The model under review builds one solid part; all positions refer to its coordinate system, in mm. Round coordinates to 2 decimals unless told otherwise and drop trailing zeros. Write each loop counter-clockwise with the first axis right and the second up, starting at its lowest first coordinate (ties: lowest second). Pieces come first, ordered by that corner, then holes. Notation, with made-up numbers: M 60.25,-7 L 92.25,-7 A29 ccw 92.25,27 Z; hole C 68.5,-27.75 d1. An arc over 180 degrees is marked long. One line per item, written item: value. Start each with the question number.
1) For P1, Ø2, axis at y = -366, z = 3, coming from the +X side, flat-tipped, find the tip position at first contact; note if it passes through.
2) Take a section at B-B, the plane z = 2.5. State how many separate pieces and enclosed holes the cut face has, and give its area (3 significant figures).
3) Take a section at A-A, the plane y = -298.5. Write out the cut boundary in (x, z), and give its area (3 significant figures).
4) Wall thickness on probe 1 along Y at (x, z) = (222.25, 3); probe 2 along Y at (x, z) = (0, 5.25); probe 3 along Y at (x, z) = (444.5, 2): over which ranges is each line inside the solid? List them lowest first.
from build123d import *

# Parameters (mm, degrees)
BOSS_EXTRUDE1_DEPTH = 6.35
SKETCH2_R           = 3.3655
CUT_EXTRUDE1_DEPTH  = 7.35
SKETCH3_R           = 3.3655
CUT_EXTRUDE2_DEPTH  = 7.35
SKETCH5_W           = 38.1
SKETCH5_H           = 82.55
CUT_EXTRUDE3_DEPTH  = 7.35
FILLET1_R           = 6.35


with BuildPart() as part:
    # Sketch1 → Boss-Extrude1 (new body)
    with BuildSketch(Plane.XY):
        Polygon((-508, 0), (508, 0), (508, -184.15), (234.95, -184.15), (234.95, -457.2), (-234.95, -457.2), (-234.95, -184.15), (-508, -184.15), align=None)
    extrude(amount=BOSS_EXTRUDE1_DEPTH)

    # Sketch2 → Cut-Extrude1 (cut, through all)
    with BuildSketch(Plane.XY.offset(6.35)):
        with Locations((0, -9.525)):
            Circle(SKETCH2_R)
        with Locations((0, -447.675)):
            Circle(SKETCH2_R)
        with Locations((222.25, -9.525)):
            Circle(SKETCH2_R)
        with Locations((222.25, -447.675)):
            Circle(SKETCH2_R)
        with Locations((444.5, -9.525)):
            Circle(SKETCH2_R)
        with Locations((-222.25, -9.525)):
            Circle(SKETCH2_R)
        with Locations((-222.25, -447.675)):
            Circle(SKETCH2_R)
        with Locations((-444.5, -9.525)):
            Circle(SKETCH2_R)
    extrude(amount=-CUT_EXTRUDE1_DEPTH, mode=Mode.SUBTRACT)

    # Sketch3 → Cut-Extrude2 (cut, through all)
    with BuildSketch(Plane.XY.offset(6.35)):
        with Locations((-460.375, -25.4)):
            Circle(SKETCH3_R)
        with Locations((-460.375, -158.75)):
            Circle(SKETCH3_R)
    cut_extrude2 = extrude(amount=-CUT_EXTRUDE2_DEPTH, mode=Mode.SUBTRACT)

    # Mirror1: Cut-Extrude2 across plane
    add(cut_extrude2.mirror(Plane(origin=(0, 0, 0), x_dir=(0, 0, 1), z_dir=(1, 0, 0))), mode=Mode.SUBTRACT)

    # Sketch5 → Cut-Extrude3 (cut, through all)
    with BuildSketch(Plane.XY.offset(6.35)):
        with Locations((-215.9, -371.475)):
            Rectangle(SKETCH5_W, SKETCH5_H)
    cut_extrude3 = extrude(amount=-CUT_EXTRUDE3_DEPTH, mode=Mode.SUBTRACT)

    # Mirror2: Cut-Extrude3 across plane
    add(cut_extrude3.mirror(Plane(origin=(0, 0, 0), x_dir=(0, 0, 1), z_dir=(1, 0, 0))), mode=Mode.SUBTRACT)

    # Fillet1
    fillet1_edges = [part.edges().sort_by_distance(p)[0] for p in [
        (234.95, -330.2, 3.175),
        (234.95, -412.75, 3.175),
        (196.85, -412.75, 3.175),
        (196.85, -330.2, 3.175),
        (-508, 0, 3.175),
        (508, 0, 3.175),
        (508, -184.15, 3.175),
        (234.95, -184.15, 3.175),
        (234.95, -457.2, 3.175),
        (-234.95, -457.2, 3.175),
        (-234.95, -184.15, 3.175),
        (-508, -184.15, 3.175),
        (-234.95, -412.75, 3.175),
        (-234.95, -330.2, 3.175),
        (-196.85, -330.2, 3.175),
        (-196.85, -412.75, 3.175),
    ]]
    fillet(fillet1_edges, radius=FILLET1_R)


solid = part.part
Checked values:
1. P1: stops at x = 196.85
2. separate pieces: 1
2. enclosed holes: 12
2. area: 309,000 mm2
3. outline: M -234.95,0 L 234.95,0 L 234.95,6.35 L -234.95,6.35 Z
3. area: 2,980 mm2
4. probe 1: y = -457.2 to -451.04, -444.31 to -412.75, -330.2 to -12.89, -6.16 to 0
4. probe 2: y = -457.2 to -451.04, -444.31 to -12.89, -6.16 to 0
4. probe 3: y = -184.15 to -12.89, -6.16 to 0
